Design review of the part built by this model. Coordinates are the model's own, in mm. Face numbers are marked on the shaded views. A direction names the side the tool comes from. Give positions to 0.01 mm unless a question says otherwise; leave off trailing zeros. Loops run counter-clockwise (first coordinate to the right, second up) from the corner with the lowest first, then second, coordinate; pieces in that order, holes last. Notation, with made-up numbers: M 80,-16.75 L 131,-16.75 A17 ccw 131,15.25 Z; hole C 63.25,38.25 d11. An arc over 180 degrees is marked long. Use one line per item in the form item = value. Start each with the question number.
from build123d import *

# Parameters (mm, degrees)
SKETCH1_W           = 228
SKETCH1_H           = 101
BOSS_EXTRUDE1_DEPTH = 5
SKETCH2_R           = 2
CUT_EXTRUDE1_DEPTH  = 250.419325635
SKETCH3_W           = 228
SKETCH3_H           = 85
BOSS_EXTRUDE2_DEPTH = 34.8
SKETCH4_W           = 19.026867748
SKETCH4_H           = 7.567504218
BOSS_EXTRUDE3_DEPTH = 2.2
FILLET1_R           = 10


with BuildPart() as part:
    # Sketch1 → Boss-Extrude1 (new body)
    with BuildSketch(Plane(origin=(0, 0, 0), x_dir=(1, 0, 0), z_dir=(0, 1, 0))):
        with Locations((114, 50.5)):
            Rectangle(SKETCH1_W, SKETCH1_H)
    extrude(amount=BOSS_EXTRUDE1_DEPTH)

    # Sketch2 → Cut-Extrude1 (cut, through all)
    with BuildSketch(Plane(origin=(0, 5, 0), x_dir=(1, 0, 0), z_dir=(0, 1, 0))):
        with Locations(Location((187.34, 97, 0), (0, 0, 270))):
            Circle(SKETCH2_R)
        with Locations(Location((187.34, 4, 0), (0, 0, 270))):
            Circle(SKETCH2_R)
        with Locations(Location((114, 97, 0), (0, 0, 270))):
            Circle(SKETCH2_R)
        with Locations(Location((40.66, 97, 0), (0, 0, 270))):
            Circle(SKETCH2_R)
        with Locations(Location((114, 4, 0), (0, 0, 90))):
            Circle(SKETCH2_R)
        with Locations(Location((40.66, 4, 0), (0, 0, 90))):
            Circle(SKETCH2_R)
    extrude(amount=-CUT_EXTRUDE1_DEPTH, mode=Mode.SUBTRACT)

    # Sketch3 → Boss-Extrude2 (add)
    with BuildSketch(Plane(origin=(0, 5, 0), x_dir=(1, 0, 0), z_dir=(0, 1, 0))):
        with Locations((114, 50.5)):
            Rectangle(SKETCH3_W, SKETCH3_H)
    extrude(amount=BOSS_EXTRUDE2_DEPTH)

    # Sketch4 → Boss-Extrude3 (add)
    with BuildSketch(Plane.ZY):
        with Locations((-40.824405321, 21.683781351)):
            Rectangle(SKETCH4_W, SKETCH4_H)
    extrude(amount=BOSS_EXTRUDE3_DEPTH)

    # Fillet1
    fillet1_edges = [part.edges().sort_by_distance(p)[0] for p in [
        (0, 2.5, 0),
    ]]
    fillet(fillet1_edges, radius=FILLET1_R)
    fillet1_2_edges = [part.edges().sort_by_distance(p)[0] for p in [
        (228, 2.5, 0),
    ]]
    fillet(fillet1_2_edges, radius=FILLET1_R)
    fillet1_3_edges = [part.edges().sort_by_distance(p)[0] for p in [
        (0, 2.5, -101),
    ]]
    fillet(fillet1_3_edges, radius=FILLET1_R)
    fillet1_4_edges = [part.edges().sort_by_distance(p)[0] for p in [
        (228, 2.5, -101),
    ]]
    fillet(fillet1_4_edges, radius=FILLET1_R)
    fillet1_5_edges = [part.edges().sort_by_distance(p)[0] for p in [
        (114, 39.8, -93),
    ]]
    fillet(fillet1_5_edges, radius=FILLET1_R)
    fillet1_6_edges = [part.edges().sort_by_distance(p)[0] for p in [
        (114, 39.8, -8),
    ]]
    fillet(fillet1_6_edges, radius=FILLET1_R)


solid = part.part
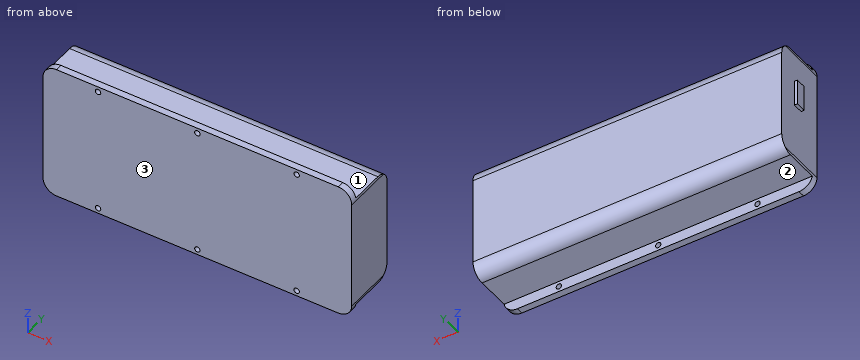
Q1. Take a section at B-B on y = 15.5. Give the boundary of the cut face in (x, z), plus the area to 3 significant figures.
Q2. Take a section at A-A on x = 49. Give the boundary of the cut face in (y, z).
Q3. Clearance check with flat-ended pins moving along their axes: pin 1 Ø4.5 at (x, z) = (40.66, -97) entering from +Y; pin 2 Ø3 at (x, z) = (40.66, -4) entering from -Y; pin 3 Ø7.5 at (x, y) = (150.5, 14) entering from -Z; pin 4 Ø1.1 at (x, z) = (-1, -42.5) entering from +Y. State where each tip first meets the part, or that it passes through.
Q4. For the marked faces 1, 2 and 3, list the 3-axis set-ups (+Z, -Z, +X, -X, +Y, -Y) from which the entire face can be reached by the end or side of a thin tool; tool diameter is ignored.
Q5. Wall thickness on probe 1 along Z at (x, y) = (187.34, 1.4); probe 2 along X at (y, z) = (1, -97); probe 3 along Z at (x, y) = (140.5, 8.5): over which ranges is each line inside the solid? List them lowest first.
Response values:
q1.outline = M 0,-91 A10 ccw 0.2,-93 L 227.8,-93 A10 ccw 228,-91 L 228,-10 A10 ccw 227.8,-8 L 0.2,-8 A10 ccw 0,-10 Z
q1.area = 19,400 mm^2
q2.outline = M 0,-101 L 5,-101 L 5,-93 L 29.8,-93 A10 ccw 39.8,-83 L 39.8,-18 A10 ccw 29.8,-8 L 5,-8 L 5,0 L 0,0 Z
q3.pin_1 = 5
q3.pin_2 = through
q3.pin_3 = -93
q3.pin_4 = 25.47
q4.face_1 = +Z, +X, -X, +Y
q4.face_2 = -Z, +X, -X, +Y
q4.face_3 = +Z, -Z, +X, -X, -Y
q5.probe_1 = -101 to -99, -95 to -6, -2 to 0
q5.probe_2 = 2 to 38.66, 42.66 to 112, 116 to 185.34, 189.34 to 226
q5.probe_3 = -93 to -8
